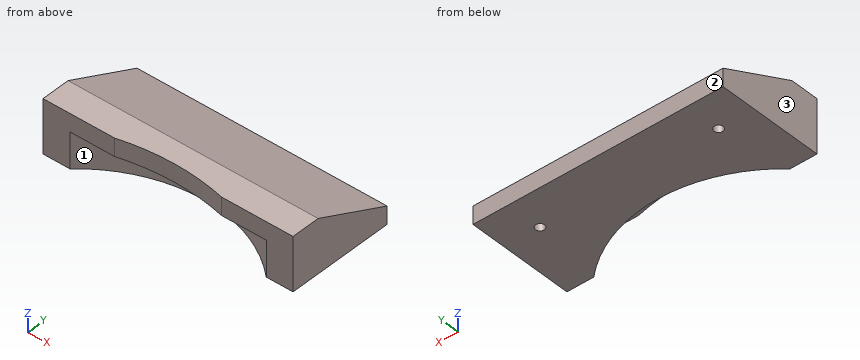
from build123d import *

# Parameters (mm, degrees)
F0_W     = 88.9
F0_H     = 38.1
F1_DEPTH = 19.05
F3_DEPTH = 88.9
F5_DEPTH = 25.4
F7_DEPTH = 12.7
F9_D     = 3.175
F9_DEPTH = 10.16
F9_TIP   = 0.9538662327


with BuildPart() as f1:
    # F0 (on Top) → F1 (new body)
    with BuildSketch(Plane.XY):
        Rectangle(F0_W, F0_H)
    extrude(amount=F1_DEPTH)

    # F2 (on face) → F3 (cut)
    with BuildSketch(Plane(origin=(-44.45, 0, 0), x_dir=(0, -1, 0), z_dir=(-1, 0, 0))):
        Polygon((-19.05, 19.05), (-19.05, 6.35), (8.89, 19.05), align=None)
    extrude(amount=-F3_DEPTH, mode=Mode.SUBTRACT)

    # F4 (on face) → F5 (cut)
    with BuildSketch(Plane.XY.offset(19.05)):
        with BuildLine():
            ThreePointArc((19.05, -19.05), (0, -16.7213844667), (-19.05, -19.05))
            Line((-19.05, -19.05), (19.05, -19.05))
        make_face()
    extrude(amount=-F5_DEPTH, mode=Mode.SUBTRACT)

    # F6 (on face) → F7 (cut)
    with BuildSketch(Plane(origin=(0, 0, 0), x_dir=(1, 0, 0), z_dir=(0, 0, -1))):
        with BuildLine():
            ThreePointArc((-34.925, 19.05), (0, 5.3458547425), (34.925, 19.05))
            Line((34.925, 19.05), (19.05, 19.05))
            ThreePointArc((19.05, 19.05), (0, 16.7213844667), (-19.05, 19.05))
            Line((-19.05, 19.05), (-34.925, 19.05))
        make_face()
    extrude(amount=-F7_DEPTH, mode=Mode.SUBTRACT)

    # F9
    with Locations(Plane(origin=(0, 0, 0), x_dir=(1, 0, 0), z_dir=(0, 0, -1))):
        with Locations((31.75, -6.35), (-31.75, -6.35)):
            Hole(F9_D / 2, depth=F9_DEPTH)
            with Locations((0, 0, -(F9_DEPTH + F9_TIP / 2))):  # 118° drill point
                Cone(0, F9_D / 2, F9_TIP, mode=Mode.SUBTRACT)


solid = f1.part
Part model, mm, in its own coordinate system. Face numbers are marked on the shaded views. Round coordinates to 2 decimals unless told otherwise and drop trailing zeros. Write each loop counter-clockwise with the first axis right and the second up, starting at its lowest first coordinate (ties: lowest second). Pieces come first, ordered by that corner, then holes. Notation, with made-up numbers: M 55,1 L 90,1 A22 cw 90,14 Z; hole C 62,30 d4. An arc over 180 degrees is marked long. Return JSON: item names as keys, results as strings. Group by question number.
(1) Saw through at D-D on y = 16.5. Write the cut outline in (x, z), then the cut area to 3 significant figures.
(2) Saw through at C-C on z = 18. Write the cut outline in (x, y), then the cut area to 3 significant figures.
(3) Drill centre lines: probe 1 along X at (y, z) = (6.35, 7.5); probe 2 along Z at (x, y) = (-21, -15.5); probe 3 along Y at (x, z) = (-31.75, 7). Where is each one in solid material? Low to high.
(4) Saw through at A-A on y = -8. Write the cut outline in (x, z).
(5) Pin check, flat tips, straight feed: pin 1 Ø3 at (y, z) = (7.5, 12.5) entering from -X; pin 2 Ø1 at (x, z) = (4.5, 7) entering from +Y; pin 3 Ø2 at (x, z) = (-28.5, 7) entering from -Y; pin 4 Ø3 at (x, z) = (-12, 8.5) entering from +Y. Stop position of each tip, or through.
(6) Saw through at B-B on x = -37. Write the cut outline in (y, z).
(7) Two-plate mould, pull along X, no slides. Class the marked faces 1, 2 and 3: +X half, -X half, draft (parallel to the pull), parting line (faces both ways), or undercut.
Returned:
{
 "1": {"outline": "M -44.45,0 L 44.45,0 L 44.45,7.51 L -44.45,7.51 Z", "area": "668 mm²"},
 "2": {"outline": "M -44.45,-19.05 L -19.05,-19.05 A79.09 cw 19.05,-19.05 L 44.45,-19.05 L 44.45,-6.58 L -44.45,-6.58 Z", "area": "1,050 mm²"},
 "3": {"probe 1": "-44.45 to -33.34, -30.16 to 30.16, 33.34 to 44.45", "probe 2": "12.7 to 19.05", "probe 3": "-16.34 to 4.76, 7.94 to 17.62"},
 "4": {"outline": "M -44.45,0 L -16.3,0 L -16.3,12.7 L 16.3,12.7 L 16.3,0 L 44.45,0 L 44.45,18.65 L -44.45,18.65 Z"},
 "5": {"pin 1": "x = -44.45", "pin 2": "y = 18.72", "pin 3": "y = -14.66", "pin 4": "y = 17.62"},
 "6": {"outline": "M -19.05,0 L 19.05,0 L 19.05,6.35 L -8.89,19.05 L -19.05,19.05 Z"},
 "7": {"face 1": "undercut", "face 2": "draft", "face 3": "-X half"}
}
